```python
from build123d import *

# Parameters (mm, degrees)
F0_W     = 139.7
F0_H     = 101.6
F1_DEPTH = 1.5875
F2_R     = 2.413
F3_DEPTH = 1.5875


with BuildPart() as f1:
    # F0 (on Front) → F1 (new body, symmetric)
    with BuildSketch(Plane.XZ):
        Rectangle(F0_W, F0_H)
    extrude(amount=F1_DEPTH, both=True)

    # F2 (on Front) → F3 (cut, symmetric)
    with BuildSketch(Plane.XZ):
        with Locations((19.05, 44.45)):
            Circle(F2_R)
        with Locations((-19.05, 44.45)):
            Circle(F2_R)
        with Locations((-63.5, 19.05)):
            Circle(F2_R)
        with Locations((-63.5, -25.4)):
            Circle(F2_R)
        with Locations((63.5, 19.05)):
            Circle(F2_R)
        with Locations((63.5, -25.4)):
            Circle(F2_R)
        with Locations((-31.75, -41.402)):
            Circle(F2_R)
        with Locations((31.75, -41.402)):
            Circle(F2_R)
    extrude(amount=F3_DEPTH, both=True, mode=Mode.SUBTRACT)


solid = f1.part
```
CAD build for the part. Positions are in the model's coordinates, mm. Round coordinates to 2 decimals unless told otherwise and drop trailing zeros. Write each loop counter-clockwise with the first axis right and the second up, starting at its lowest first coordinate (ties: lowest second). Pieces come first, ordered by that corner, then holes. Notation, with made-up numbers: M -24,70 L 13,70 A25 ccw 13,103 Z; hole C 54,-25.75 d8. An arc over 180 degrees is marked long. One line per question, with ' | ' between items.
1. Probe L1, parallel to Z at x = 63.5, y = -0.6; L2, parallel to Z at x = 31.75, y = 0.5 (3 decimals); L3, parallel to X at y = 1.4, z = 42.5. List the from-to ranges inside material, lowest first. Write a range as from..to.
Working result:
L1: -50.8..-27.81, -22.99..16.64, 21.46..50.8 | L2: -50.8..-43.815, -38.989..50.8 | L3: -69.85..-20.47, -17.63..17.63, 20.47..69.85
2. Cut at A-A on x = 19.05. Write the cut outline in (y, z).
Working result:
outline: M -1.59,-50.8 L 1.59,-50.8 L 1.59,42.04 L -1.59,42.04 Z; M -1.59,46.86 L 1.59,46.86 L 1.59,50.8 L -1.59,50.8 Z
3. Cut at B-B on z = 44.45. Write the cut outline in (x, y), and give its area (3 significant figures).
Working result:
outline: M -69.85,-1.59 L -21.46,-1.59 L -21.46,1.59 L -69.85,1.59 Z; M -16.64,-1.59 L 16.64,-1.59 L 16.64,1.59 L -16.64,1.59 Z; M 21.46,-1.59 L 69.85,-1.59 L 69.85,1.59 L 21.46,1.59 Z | area: 413 mm2
4. Mould opens along X. For faces 1 (the flat face through (-69.85, 0, -1)), 2 (the cylindrical face through (32.863, -0.022, -43.543)), 3 (the flat face through (-1, -1.588, 1)) say: pulls with the +X half, pulls with the -X half, needs draft (parallel to the pull), parting line crosses it, or undercut.
Working result:
face 1: pulls with the -X half | face 2: undercut | face 3: needs draft
5. Cut at C-C on x = -63.5. Write the cut outline in (y, z).
Working result:
outline: M -1.59,-50.8 L 1.59,-50.8 L 1.59,-27.81 L -1.59,-27.81 Z; M -1.59,-22.99 L 1.59,-22.99 L 1.59,16.64 L -1.59,16.64 Z; M -1.59,21.46 L 1.59,21.46 L 1.59,50.8 L -1.59,50.8 Z
